from build123d import *

# Parameters (mm, degrees)
F0_W     = 135
F0_H     = 150
F1_DEPTH = 10
F2_R     = 5
F3_DEPTH = 5


with BuildPart() as f1:
    # F0 (on Front) → F1 (new body)
    with BuildSketch(Plane.XZ):
        Rectangle(F0_W, F0_H)
    extrude(amount=-F1_DEPTH)

    # F2 (on face) → F3 (join)
    with BuildSketch(Plane.XZ):
        with Locations((-20, -41.855509)):
            Circle(F2_R)
        with Locations((20, -41.855509)):
            Circle(F2_R)
        with Locations((20, 6.144491)):
            Circle(F2_R)
        with Locations((-26, 6.144491)):
            Circle(F2_R)
        with Locations((-26, 54.144491)):
            Circle(F2_R)
        with Locations((20, 54.144491)):
            Circle(F2_R)
    extrude(amount=F3_DEPTH)


solid = f1.part
Input: part model. Units: mm. Frame: model coordinates. A direction names the side the tool comes from. Round coordinates to 2 decimals unless told otherwise and drop trailing zeros. Order: outer loops, then holes, each group sorted by start corner. A loop starts at its lowest first (then second) coordinate and runs counter-clockwise, first axis right, second up. Notation, with made-up numbers: (-10, -14.5) - (3, -14.5) arc R21 cw to (3, 7.5) - close; hole circle Ø11 at (-12.5, -3.5). An arc over 180 degrees is marked (long way). Answer as a JSON object with one key per item and string values. Group by question number.
(1) Cut plane B-B (y = -3.25). Return loops of the section in (x, z).
(2) Cut plane D-D (z = 56). Return loops of the section in (x, y), then the cut area to 3 significant figures.
(3) Pin query (flat end, axial travel): P1, Ø8, axis at x = 4, z = 55, coming from the -Y side. Return the tip coordinate at first contact, or that it passes through.
(4) Reachability of faces 1 (the face through (19.349, -2.465, -36.898)), 2 (the face through (20, -5, 54)) from +Z, -Z, +X, -X, +Y, -Y: full face, straight path, thin tool, end or side. Return the list, or none.
(5) Cut plane C-C (z = -27). Return loops of the section in (x, y).
(6) Draft query along Z for faces 3 (the face through (-1, 5, 75)), 4 (the face through (20, -5, 6)), 5 (the face through (19.349, -2.465, 11.102)), 6 (the face through (-20.651, -2.465, -36.898)). Return one class per face: released by +Z, released by -Z, zero draft, split by the parting line, or undercut.
(7) Cut plane A-A (x = 20). Return loops of the section in (y, z), then the cut area to 3 significant figures.
(8) Material intervals for probe 1 along Y at (x, z) = (54.5, -31); probe 2 along X at (y, z) = (-0.5, -45), sorted ascending. Write a range as from..to.
Here are the results:
{
 "1": {"outline": "circle Ø10 at (-26, 6.14); circle Ø10 at (-26, 54.14); circle Ø10 at (-20, -41.86); circle Ø10 at (20, -41.86); circle Ø10 at (20, 6.14); circle Ø10 at (20, 54.14)"},
 "2": {"outline": "(-67.5, 0) - (-30.64, 0) - (-30.64, -5) - (-21.36, -5) - (-21.36, 0) - (15.36, 0) - (15.36, -5) - (24.64, -5) - (24.64, 0) - (67.5, 0) - (67.5, 10) - (-67.5, 10) - close", "area": "1,440 mm^2"},
 "3": {"P1": "stops at y = 0"},
 "4": {"face 1": "-Y", "face 2": "+Z, -Z, +X, -X, -Y"},
 "5": {"outline": "(-67.5, 0) - (67.5, 0) - (67.5, 10) - (-67.5, 10) - close"},
 "6": {"face 3": "released by +Z", "face 4": "zero draft", "face 5": "undercut", "face 6": "undercut"},
 "7": {"outline": "(-5, -46.86) - (0, -46.86) - (0, -75) - (10, -75) - (10, 75) - (0, 75) - (0, 59.14) - (-5, 59.14) - (-5, 49.14) - (0, 49.14) - (0, 11.14) - (-5, 11.14) - (-5, 1.14) - (0, 1.14) - (0, -36.86) - (-5, -36.86) - close", "area": "1,650 mm^2"},
 "8": {"probe 1": "y = 0..10", "probe 2": "x = -23.89..-16.11, 16.11..23.89"}
}
